from build123d import *

# Parameters (mm, degrees)
BOSS_EXTRUDE1_DEPTH = 23.78
BOSS_EXTRUDE2_DEPTH = 6


with BuildPart() as part:
    # Sketch3 → Boss-Extrude1 (new body)
    with BuildSketch(Plane(origin=(48.18, 0, 0), x_dir=(0, 0, -1), z_dir=(1, 0, 0))):
        with BuildLine():
            Line((17.45, 13.265), (9, 13.265))
            Line((9, 13.265), (9, -9))
            Line((9, -9), (-13.265, -9))
            Line((-13.265, -9), (-13.265, -17.45))
            ThreePointArc((-13.265, -17.45), (15.499398779, -15.499398779), (17.45, 13.265))
        make_face()
    extrude(amount=-BOSS_EXTRUDE1_DEPTH)

    # Sketch4 → Boss-Extrude2 (add)
    with BuildSketch(Plane(origin=(36.29, 0, 0), x_dir=(0, 0, -1), z_dir=(1, 0, 0))):
        with BuildLine():
            Line((3.984372706, -16.433233831), (4.643364687, -9))
            Line((4.643364687, -9), (7.595, -9))
            ThreePointArc((7.595, -9), (11.734437034, -0.993485028), (9, 7.595))
            Line((9, 7.595), (-0.841557906, 5.366649873))
            Line((-0.841557906, 5.366649873), (-16.433233831, 3.984372706))
            ThreePointArc((-16.433233831, 3.984372706), (-19.030672408, 2.700654058), (-20.08, 0))
            ThreePointArc((-20.08, 0), (-14.198704166, -14.198704166), (0, -20.08))
            ThreePointArc((0, -20.08), (2.700654058, -19.030672408), (3.984372706, -16.433233831))
        make_face()
    extrude(amount=-BOSS_EXTRUDE2_DEPTH)


solid = part.part
Build history of the part. All positions in model axes, mm. Round coordinates to 2 decimals unless told otherwise and drop trailing zeros. Write each loop counter-clockwise with the first axis right and the second up, starting at its lowest first coordinate (ties: lowest second). Pieces come first, ordered by that corner, then holes. Notation, with made-up numbers: (37, -37) -> (95, -37) arc R24 cw to (95, -2) -> close; hole circle Ø10 at (25.25, 24). An arc over 180 degrees is marked (long way). Use one line per item in the form item = value.
Q1. Two-plate mould, pull along Z, no slides. Class faces 1 (the flat face through (24.4, -12, -8)), 2 (the cylindrical face through (33.332, -8.337, -8.317)), 3 (the flat face through (33.332, 6.496, -4.148)): released by +Z, released by -Z, zero draft, split by the parting line, or undercut.
Conclusion:
face_1 = zero draft
face_2 = undercut
face_3 = released by +Z
Q2. Drop flat-ended pins along their axis: P1, Ø12, axis at x = 33, y = 9.5, coming from the +Z side; P2, Ø6.5, axis at x = 31.5, z = -2, coming from the +Y side; P3, Ø1.5, axis at x = 45, z = 8.5, coming from the +Y side. Give the stop position or say it passes through.
Conclusion:
P1 = 18.02
P2 = 6.75
P3 = -9
Q3. Band-saw the part on B-B, the plane x = 41. Write the cut outline in (y, z) (3 decimals), then the cut area to 3 significant figures.
Conclusion:
outline = (-17.45, 13.265) arc R21.919 ccw to (13.265, -17.45) -> (13.265, -9) -> (-9, -9) -> (-9, 13.265) -> close
area = 601 mm²
Q4. Drill centre lines: L1, parallel to X at y = 2, z = -3.5; L2, parallel to Y at x = 35.5, z = -8.5; L3, parallel to Z at x = 29, y = -17.5. Where is each one in solid material? Low to high.
Conclusion:
L1 = 30.29 to 36.29
L2 = -20.2 to -9, -8.15 to 7.48
L3 = -13.2 to 13.2
Q5. Band-saw the part on C-C, the plane y = -6. Write the cut outline in (x, z), then the cut area to 3 significant figures.
Conclusion:
outline = (24.4, -21.08) -> (48.18, -21.08) -> (48.18, -9) -> (36.29, -9) -> (36.29, 19.16) -> (30.29, 19.16) -> (30.29, -9) -> (24.4, -9) -> close
area = 456 mm²
Q6. Band-saw the part on D-D, the plane z = 12. Write the cut outline in (x, y), then the cut area to 3 significant figures.
Conclusion:
outline = (24.4, -18.34) -> (48.18, -18.34) -> (48.18, -9) -> (36.29, -9) -> (36.29, 4.38) -> (30.29, 4.38) -> (30.29, -9) -> (24.4, -9) -> close
area = 302 mm²
Q7. Band-saw the part on A-A, the plane x = 32.5. Write the cut outline in (y, z) (3 decimals), then the cut area to 3 significant figures.
Conclusion:
outline = (-17.45, 13.265) arc R21.919 ccw to (13.265, -17.45) -> (13.265, -9) -> (7.595, -9) -> (5.367, 0.842) -> (3.984, 16.433) arc R4 ccw to (0, 20.08) arc R20.08 ccw to (-15.075, 13.265) -> close; hole (-9, -9) -> (-7.595, -9) arc R11.776 cw to (-9, -7.595) -> close
area = 1,020 mm²
